Could you check a few things on this model? Use its own coordinates, in mm. A direction names the side the tool comes from. Give positions to 0.01 mm unless a question says otherwise; leave off trailing zeros. Loops run counter-clockwise (first coordinate to the right, second up) from the corner with the lowest first, then second, coordinate; pieces in that order, holes last. Notation, with made-up numbers: (-35.75, 80) -> (3.25, 80) arc R17 cw to (3.25, 111) -> close; hole circle Ø6 at (-25.75, 28.25). An arc over 180 degrees is marked (long way). Write each question's results on one line, items separated by ' | '. Start each with the question number.
Q1. If we section it at B-B, the plane z = -467: List the corners of the cut face in (x, y) for me.
Q2. Will these pins go through, and if not, where does the flat tip stop? P1, Ø12, axis at x = 14.5, z = -129.5, coming from the +Y side; P2, Ø12, axis at x = 72.5, y = 602.5, coming from the -Z side.
Q3. If I drill on line 1 along Z through (x, y) = (105, 757.5); line 2 along Y through (x, z) = (109, -789.5), over which ranges is the centre line in solid material (lowest first)?
Q4. If we section it at C-C, the plane y = 532: List the corners of the cut face in (x, z) for me, plus the area to 3 significant figures.
Q5. If we section it at D-D, the plane x = 92: List the corners of the cut face in (y, z) for me.
Q6. If we section it at A-A, the plane x = 17: List the corners of the cut face in (y, z) for me, plus the area to 3 significant figures.
Q7. Which directions (+Z, -Z, +X, -X, +Y, -Y) give clear straight access to the entire face, cutting with the end or side of a thin tool? Please do faces 1 (the face through (57, 511, 0)), 2 (the face through (94.72, -2.96, -835.63)).
from build123d import *
from OCP.BRepFilletAPI import BRepFilletAPI_MakeChamfer

# Parameters (mm, degrees)
SM_BASE_FLANGE_1_DEPTH = 115
CHAMFER_1_SIZE         = 90
CHAMFER_1_SIZE2        = 40
CHAMFER_2_SIZE         = 40
CHAMFER_2_SIZE2        = 90


# Sheet-metal steps are written as plain solids
with BuildPart() as part:
    # Sketch 1 → 基体-法兰1 (new body)
    with BuildSketch(Plane(origin=(0, 0, 0), x_dir=(0, 0, -1), z_dir=(1, 0, 0))):
        with BuildLine():
            Line((0, 980), (0, 29.485281374))
            ThreePointArc((0, 29.485281374), (0.456722805, 27.18918078), (1.757359313, 25.242640687))
            Line((1.757359313, 25.242640687), (25.242640687, 1.757359313))
            ThreePointArc((25.242640687, 1.757359313), (27.18918078, 0.456722805), (29.485281374, 0))
            Line((29.485281374, 0), (880, 0))
            Line((880, 0), (880, -6))
            Line((880, -6), (29.485281374, -6))
            ThreePointArc((29.485281374, -6), (24.893080186, -5.08655439), (21, -2.485281374))
            Line((21, -2.485281374), (-2.485281374, 21))
            ThreePointArc((-2.485281374, 21), (-5.08655439, 24.893080186), (-6, 29.485281374))
            Line((-6, 29.485281374), (-6, 980))
            Line((-6, 980), (0, 980))
        make_face()
    extrude(amount=SM_BASE_FLANGE_1_DEPTH)

    # 倒角1
    chamfer_1_edges = [part.edges().sort_by_distance(p)[0] for p in [
        (115, 980, 3),
        (115, -3, -880),
    ]]
    chamfer_1_side = [part.faces().sort_by_distance(p)[0] for p in [
        (115, 25.400361972, 3.861867822),
    ]]
    chamfer(chamfer_1_edges, length=CHAMFER_1_SIZE, length2=CHAMFER_1_SIZE2, reference=chamfer_1_side[0])

    # 倒角2: one chamfer whose edges measure the first distance from different faces: ONE call of the kernel's chamfer builder (chamfer() names one face for all edges)
    chamfer_2_edges_1 = [part.edges().sort_by_distance(p)[0] for p in [
        (0, 980, 3),
    ]]
    chamfer_2_side_1 = [part.faces().sort_by_distance(p)[0] for p in [
        (37.5, 980, 3),
    ]]
    chamfer_2_edges_2 = [part.edges().sort_by_distance(p)[0] for p in [
        (0, -3, -880),
    ]]
    chamfer_2_side_2 = [part.faces().sort_by_distance(p)[0] for p in [
        (37.5, -3, -880),
    ]]
    chamfer_2 = BRepFilletAPI_MakeChamfer(part.part.solid().wrapped)
    for e in chamfer_2_edges_1:
        chamfer_2.Add(CHAMFER_2_SIZE, CHAMFER_2_SIZE2, e.wrapped, chamfer_2_side_1[0].wrapped)  # the first distance lies on this face
    for e in chamfer_2_edges_2:
        chamfer_2.Add(CHAMFER_2_SIZE, CHAMFER_2_SIZE2, e.wrapped, chamfer_2_side_2[0].wrapped)  # the first distance lies on this face
    add(Compound.cast(chamfer_2.Shape()), mode=Mode.REPLACE)


solid = part.part
Final values:
1) outline: (0, -6) -> (115, -6) -> (115, 0) -> (0, 0) -> close
2) P1: stops at y = 0 | P2: stops at z = 0
3) line 1: z = 0 to 6 | line 2: y = -6 to 0
4) outline: (0, 0) -> (115, 0) -> (115, 6) -> (0, 6) -> close | area: 690 mm²
5) outline: (-6, -841.75) -> (0, -841.75) -> (0, -29.49) arc R6 cw to (1.76, -25.24) -> (25.24, -1.76) arc R6 cw to (29.49, 0) -> (941.75, 0) -> (941.75, 6) -> (29.49, 6) arc R12 ccw to (21, 2.49) -> (-2.49, -21) arc R12 ccw to (-6, -29.49) -> close
6) outline: (-6, -828.25) -> (0, -828.25) -> (0, -29.49) arc R6 cw to (1.76, -25.24) -> (25.24, -1.76) arc R6 cw to (29.49, 0) -> (928.25, 0) -> (928.25, 6) -> (29.49, 6) arc R12 ccw to (21, 2.49) -> (-2.49, -21) arc R12 ccw to (-6, -29.49) -> close | area: 10,500 mm²
7) face 1: -Z, +X, -X, +Y | face 2: -Z, +X, +Y, -Y
